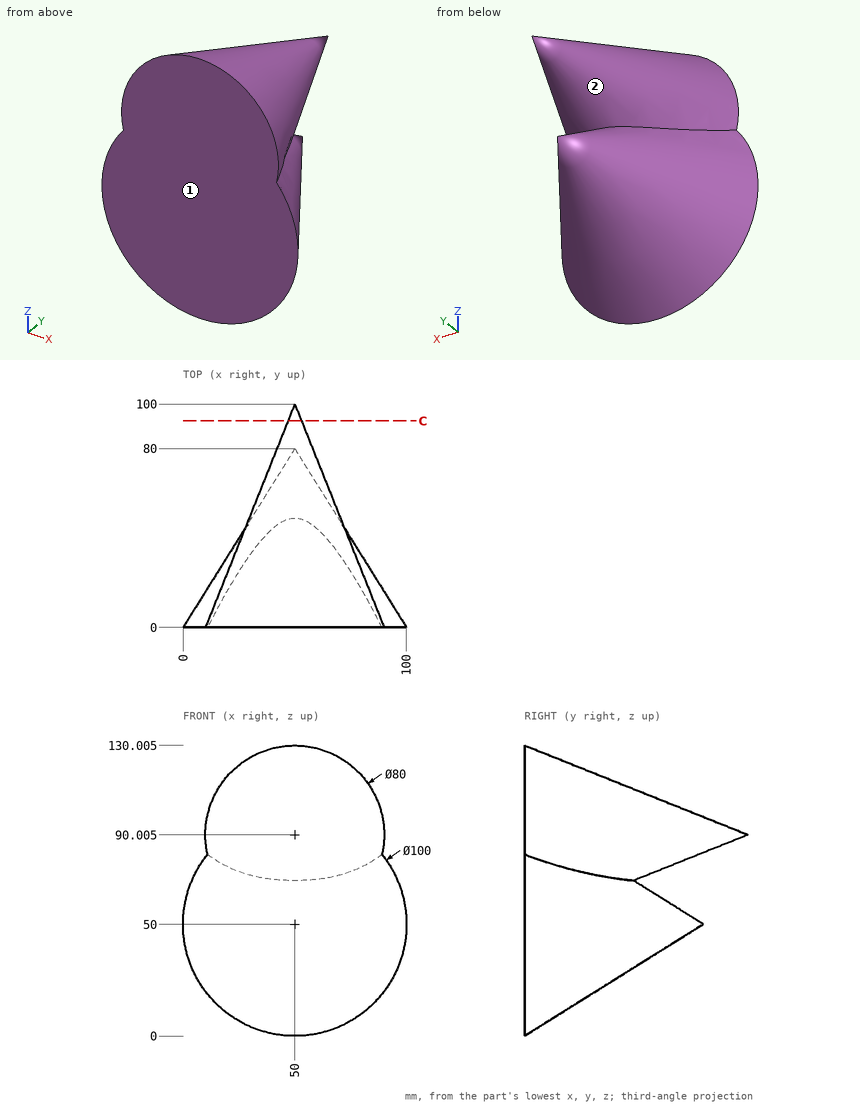
Design review of the part shown in the three views and the two pictorial views. Dimensions are in mm from the part's minimum x, y and z. Coordinates: 2 decimals unless noted, no trailing zeros. Write each loop counter-clockwise with the first axis right and the second up, starting at its lowest first coordinate (ties: lowest second). Pieces come first, ordered by that corner, then holes.
1) To check wall thickness, follow probe 1 along Z at (x, y) = (49.5, 68) (1 decimal); probe 2 along Y at (x, z) = (62, 48) (1 decimal); probe 3 along Y at (x, z) = (12.5, 47.5) (1 decimal). State the ranges of each line that lie inside material, in increasing order.
2) We need section C-C on y = 92.5. State the section outline as (x, z) points (1 decimal), then the cut area to 3 significant figures.
3) Clearance check with flat-ended pins moving along their axes: pin 1 Ø12 at (y, z) = (38, 76.5) entering from +X; pin 2 Ø6 at (x, z) = (22.5, 15.5) entering from +Y; pin 3 Ø12 at (y, z) = (48, 70) entering from -X (1 decimal). State where each tip first meets the part, or that it passes through.
4) The part is to be moulded in two halves that separate along Z. For the marked faces 1 and 2, say which applies: pulls with the +Z half, pulls with the -Z half, needs draft (parallel to the pull), parting line crosses it, or undercut.
Answer list:
1. probe 1: z = 42.5 to 57.5, 77.2 to 102.8
1. probe 2: y = 0 to 60.5
1. probe 3: y = 0 to 19.9
2. outline: circle Ø6 at (50, 90)
2. area: 28.3 mm2
3. pin 1: stops at x = 74.83
3. pin 2: stops at y = 14.21
3. pin 3: stops at x = 33.7
4. face 1: needs draft
4. face 2: undercut
